from build123d import *

# Parameters (mm, degrees)
FILLET_1_R        = 0.25
SKETCH_2_W        = 2
SKETCH_2_H        = 0.5
SWEEP_1_PROFILE_R = 0.25


with BuildPart() as part:
    # 草图1 → 旋转2 (revolve)
    with BuildSketch(Plane.XY, mode=Mode.PRIVATE) as revolve_2_sk:
        Polygon((-12, 0), (-12, 4), (-10, 4), (-10, 3.25), (10, 3.25), (10, 4), (12, 4), (12, 0), align=None)
    revolve(revolve_2_sk.sketch.rotate(Axis((-12, 0, 0), (1, 0, 0)), 180), axis=Axis((-12, 0, 0), (1, 0, 0)))

    # 圆角1
    fillet_1_edges = [part.edges().sort_by_distance(p)[0] for p in [
        (-10, 4, 0),
        (-10, 3.25, 0),
        (10, 3.25, 0),
        (10, 4, 0),
    ]]
    fillet(fillet_1_edges, radius=FILLET_1_R)

    # 草图2 → 旋转3 (revolve)
    with BuildSketch(Plane.XY, mode=Mode.PRIVATE) as revolve_3_sk:
        with Locations((3, 3.25)):
            Rectangle(SKETCH_2_W, SKETCH_2_H)
        with Locations((0, 3.25)):
            Rectangle(SKETCH_2_W, SKETCH_2_H)
        with Locations((6, 3.25)):
            Rectangle(SKETCH_2_W, SKETCH_2_H)
        with Locations((-3, 3.25)):
            Rectangle(SKETCH_2_W, SKETCH_2_H)
        with Locations((-6, 3.25)):
            Rectangle(SKETCH_2_W, SKETCH_2_H)
    revolve(revolve_3_sk.sketch.rotate(Axis((-1000, 0, 0), (1, 0, 0)), 90), axis=Axis((-1000, 0, 0), (1, 0, 0)))

    # 扫描1: sweep along a path in 草图3
    with BuildLine(Plane.XY) as sweep_1_path:
        Line((-12, 0), (-13, 0))
        Line((-13, 0), (-13, -7))
    # 扫描1 profile (on start of the path) → 扫描1 (sweep)
    with BuildSketch(Plane(origin=(-12, 0, 0), x_dir=(0, -1, 0), z_dir=(-1, 0, 0))):
        Circle(SWEEP_1_PROFILE_R)
    sweep_1 = sweep(path=sweep_1_path.line, transition=Transition.RIGHT)

    # 镜向1: 扫描1 across plane
    add(sweep_1.mirror(Plane(origin=(0, 0, 0), x_dir=(0, 0, 1), z_dir=(1, 0, 0))))


solid = part.part
Geometry: final body of the model. Coordinates: model frame, mm. Round coordinates to 2 decimals unless told otherwise and drop trailing zeros. Order: outer loops, then holes, each group sorted by start corner. A loop starts at its lowest first (then second) coordinate and runs counter-clockwise, first axis right, second up. Notation, with made-up numbers: (-0.5, 50) -> (29.5, 50) arc R19 ccw to (29.5, 85) -> close; hole circle Ø7 at (49, 72.25). An arc over 180 degrees is marked (long way). Put each result on its own line as item: value. Start each with the question number.
Q1. Section A-A on x = 6.5. Return the cut outline in (y, z), and give its area (3 significant figures).
Q2. First-contact query: pin 1 (2 mm diameter, centred on y = 0, z = -0.5, fed in from -X); pin 2 (3 mm diameter, centred on x = 5, z = 1, fed in from -Y); pin 3 (2 mm diameter, centred on y = -1, z = 1.5, fed in from +X); pin 4 (1.5 mm diameter, centred on x = -4.5, y = 1, fed in from -Z). Flat tips, straight axial feed; report the tip coordinate or a pass-through.
Q3. Section B-B on y = -2.5. Give the number of separate pieces and of enclosed holes in the cut face, and give its area (3 significant figures).
Q4. Line query: probe 1 along X at (y, z) = (-0.75, 3); probe 2 along Z at (x, y) = (-9.25, 0); probe 3 along Z at (x, y) = (0.75, -0.5). Output: solid intervals per line, ascending.
Q5. Section C-C on x = 13. Return the cut outline in (y, z).
Ans:
1. outline: circle Ø7 at (0, 0)
1. area: 38.5 mm2
2. pin 1: stops at x = -13.25
2. pin 2: stops at y = -3.5
2. pin 3: stops at x = 12
2. pin 4: stops at z = -3.47
3. separate pieces: 3
3. enclosed holes: 0
3. area: 116 mm2
4. probe 1: x = -12 to 12
4. probe 2: z = -3.25 to 3.25
4. probe 3: z = -3.46 to 3.46
5. outline: (-7, -0.25) -> (0, -0.25) arc R0.25 ccw to (0, 0.25) -> (-7, 0.25) -> close
